from build123d import *

# Parameters (mm, degrees)
F0_W     = 90
F0_H     = 70
F1_DEPTH = 90
F2_R     = 37
F3_DEPTH = 70
F4_R     = 5
F5_DEPTH = 9
F6_R     = 7
F8_DEPTH = 55


with BuildPart() as f1:
    # F0 (on Top) → F1 (new body)
    with BuildSketch(Plane.XY):
        Rectangle(F0_W, F0_H)
    extrude(amount=F1_DEPTH)

    # F2 (on face) → F3 (cut)
    with BuildSketch(Plane.XZ.offset(35)):
        with Locations((0, 45.5)):
            Circle(F2_R)
    extrude(amount=-F3_DEPTH, mode=Mode.SUBTRACT)

    # F4 (on face) → F5 (cut)
    with BuildSketch(Plane(origin=(0, 0, 0), x_dir=(1, 0, 0), z_dir=(0, 0, -1))):
        with Locations((-35, 25)):
            Circle(F4_R)
        with Locations((-35, -25)):
            Circle(F4_R)
        with Locations((25, 25)):
            Circle(F4_R)
        with Locations((25, -25)):
            Circle(F4_R)
    extrude(amount=-F5_DEPTH, mode=Mode.SUBTRACT)

    # F6
    f6_edges = [f1.edges().sort_by_distance(p)[0] for p in [
        (0, -35, 90),
        (45, 0, 90),
        (-45, 0, 90),
        (45, -35, 45),
        (-45, -35, 45),
    ]]
    fillet(f6_edges, radius=F6_R)

    # F7 (on face) → F8 (cut)
    with BuildSketch(Plane(origin=(0, 35, 0), x_dir=(-1, 0, 0), z_dir=(0, 1, 0))):
        with BuildLine():
            ThreePointArc((-36.9695820912, 44), (-37, 45.5), (-36.9695820912, 47))
            Line((-36.9695820912, 47), (-41.9695820912, 47))
            Line((-41.9695820912, 47), (-41.9695820912, 45.5))
            Line((-41.9695820912, 45.5), (-41.9695820912, 44))
            Line((-41.9695820912, 44), (-36.9695820912, 44))
        make_face()
        with BuildLine():
            Line((41.9695820912, 47), (36.9695820912, 47))
            ThreePointArc((36.9695820912, 47), (36.9923947412, 46.2501541923), (37, 45.5))
            ThreePointArc((37, 45.5), (36.9923947412, 44.7498458077), (36.9695820912, 44))
            Line((36.9695820912, 44), (41.9695820912, 44))
            Line((41.9695820912, 44), (41.9695820912, 45.5))
            Line((41.9695820912, 45.5), (41.9695820912, 47))
        make_face()
    extrude(amount=-F8_DEPTH, mode=Mode.SUBTRACT)


solid = f1.part
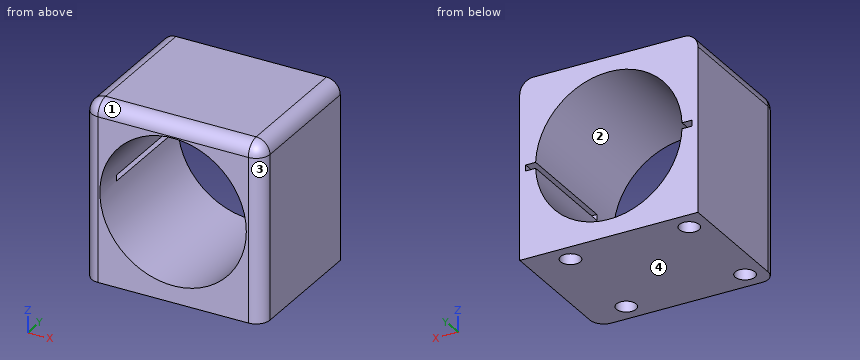
Read the model definition and answer for the solid it produces. Units are mm, in the model's axes. Face numbers are marked on the shaded views. Round coordinates to 2 decimals unless told otherwise and drop trailing zeros. Write each loop counter-clockwise with the first axis right and the second up, starting at its lowest first coordinate (ties: lowest second). Pieces come first, ordered by that corner, then holes.
1. Straight lines are drawn through the part: L1, parallel to X at y = 25, z = 4.5; L2, parallel to Y at x = 25, z = 5; L3, parallel to X at y = 13, z = 45. For each, find the intervals that lie inside material, in ascending order.
2. The part is cut by section A-A, the plane y = -1. Determine the outline of the cut face in (x, z).
3. Given pin 1 Ø6 at (x, y) = (-35, -25) entering from -Z; pin 2 Ø12 at (x, z) = (25.5, 56) entering from +Y, each flat-ended and moving along its own axis, determine where each tip first touches the part or whether it passes through.
4. Determine the mould class of the marked faces 1, 2, 3 and 4 for opening direction Z: pulls with the +Z half, pulls with the -Z half, needs draft (parallel to the pull), parting line crosses it, or undercut.
5. The part is cut by section D-D, the plane x = -35. Determine the outline of the cut face in (y, z).
6. The part is cut by section B-B, the plane z = 45.5. Determine the outline of the cut face in (x, y), then the cut area to 3 significant figures.
7. The part is cut by section C-C, the plane x = 0. Determine the outline of the cut face in (y, z), then the cut area to 3 significant figures.
Values:
1. L1: x = -45 to -40, -30 to 20, 30 to 45
1. L2: y = -35 to -30, -20 to 20, 30 to 35
1. L3: x = -45 to -41.97, 41.97 to 45
2. outline: (-45, 0) - (45, 0) - (45, 83) arc R7 ccw to (38, 90) - (-38, 90) arc R7 ccw to (-45, 83) - close; hole (-41.97, 44) - (-36.97, 44) arc R37 ccw to (36.97, 44) - (41.97, 44) - (41.97, 47) - (36.97, 47) arc R37 ccw to (-36.97, 47) - (-41.97, 47) - close
3. pin 1: stops at z = 9
3. pin 2: passes through
4. face 1: pulls with the +Z half
4. face 2: undercut
4. face 3: needs draft
4. face 4: pulls with the -Z half
5. outline: (-35, 0) - (-30, 0) - (-30, 9) - (-20, 9) - (-20, 0) - (20, 0) - (20, 9) - (30, 9) - (30, 0) - (35, 0) - (35, 33.5) - (-35, 33.5) - close; (-35, 57.5) - (35, 57.5) - (35, 90) - (-28, 90) arc R7 ccw to (-35, 83) - close
6. outline: (-45, -28) arc R7 ccw to (-38, -35) - (-37, -35) - (-37, -20) - (-41.97, -20) - (-41.97, 35) - (-45, 35) - close; (37, -35) - (38, -35) arc R7 ccw to (45, -28) - (45, 35) - (41.97, 35) - (41.97, -20) - (37, -20) - close
6. area: 552 mm2
7. outline: (-35, 0) - (35, 0) - (35, 8.5) - (-35, 8.5) - close; (-35, 82.5) - (35, 82.5) - (35, 90) - (-28, 90) arc R7 ccw to (-35, 83) - close
7. area: 1,110 mm2
